```python
from build123d import *

# Parameters (mm, degrees)
F0_W     = 89.4973501563
F0_H     = 37.3169183731
F1_DEPTH = 76.2
F2_R     = 5.08
F3_SIZE  = 25.4
F4_T     = -2.54
F6_D     = 6.35


# Not quite as in the source:
# - a shell that OpenCascade refuses in one call is made with other operations: the cavity is built on its own and cut out


with BuildPart() as f1:
    # F0 (on Front) → F1 (new body)
    with BuildSketch(Plane.XZ):
        with Locations((0.0334233046, 18.6584591866)):
            Rectangle(F0_W, F0_H)
    extrude(amount=F1_DEPTH)

    # F2
    f2_edges = [f1.edges().sort_by_distance(p)[0] for p in [
        (44.782098, -38.1, 37.316918),
        (0.033423, -76.2, 37.316918),
        (-44.715252, -38.1, 37.316918),
        (0.033423, 0, 37.316918),
    ]]
    fillet(f2_edges, radius=F2_R)

    # F3
    f3_edges = [f1.edges().sort_by_distance(p)[0] for p in [
        (-44.715252, -38.1, 0),
        (0.033423, 0, 0),
        (44.782098, -38.1, 0),
        (0.033423, -76.2, 0),
    ]]
    chamfer(f3_edges, length=F3_SIZE)

    # F4: a shell. OpenCascade refuses it in one call, so the cavity is built on its own and cut out:
    # the body offset inwards by the wall thickness, plus a prism from it out through each open face.
    f4_core = offset(f1.part, amount=F4_T, mode=Mode.PRIVATE)
    f4_exits = [f4_core.faces().sort_by_distance(p)[0] for p in [
        (0.033423, -38.1, 34.776918),
    ]]
    add(f4_core, mode=Mode.SUBTRACT)
    extrude(f4_exits, amount=-F4_T, mode=Mode.SUBTRACT)

    # F6 (through all)
    with Locations(Plane.XY.offset(2.54)):
        with Locations((0.0334233046, -40.5182316899)):
            Hole(F6_D / 2)


solid = f1.part
```
Geometry check sheet. Reference: the model listing, model coordinates, mm. A direction names the side the tool comes from. Give positions to 0.01 mm unless a question says otherwise; leave off trailing zeros. Order: outer loops, then holes, each group sorted by start corner. A loop starts at its lowest first (then second) coordinate and runs counter-clockwise, first axis right, second up. Notation, with made-up numbers: (67, 15.5) - (93, 15.5) arc R27 ccw to (93, 32.5) - close; hole circle Ø8 at (-3.75, -0.5). An arc over 180 degrees is marked (long way). Write item = value, one per line. Start each with the question number.
1) Section check B-B (z = 5). Enter the section's corners in (x, y).
2) Section check D-D (z = 17). Enter the section's corners in (x, y).
3) Section check C-C (y = -67). Enter the section's corners in (x, z).
4) Gauge pin test, flat ends, axial feed: pin 1 Ø6 at (x, z) = (9, 12) entering from -Y; pin 2 Ø1 at (y, z) = (-50.5, 8.5) entering from +X; pin 3 Ø1.3 at (y, z) = (-25.5, 35.5) entering from +X; pin 4 Ø5 at (x, y) = (0.03, -40.52) entering from +Z. Record the tip position at first contact, or that the pin passes through.
5) Draft check along X on faces 1 (the flat face through (42.242, -38, 29)), 2 (the cylindrical face through (43.333, -38.633, 35.789)), 3 (the flat face through (-34.66, -37.567, 15.344)). Enter one of: released by +X, released by -X, zero draft, split by the parting line, or undercut.
6) Access from +Z, -Z, +X, -X, +Y, -Y to the whole of each face (thin tool, end or side, straight path). Record for faces 4 (the cylindrical face through (-41.451, -38.598, 34.013)), 5 (the flat face through (-0.6, -66.5, 15.7)), 6 (the flat face through (0, -35, 2.54)).
7) Scan lines: L1, parallel to X at y = -32.5, z = 29.5; L2, parallel to Y at x = 36, z = 27; L3, parallel to Z at x = -3.5, y = -34. Record each from-to range of solid material in increasing order.
8) Section check A-A (x = -16.5). Enter the section's corners in (y, z), then the cut area to 3 significant figures.
Geometry check:
q1.outline = (-24.32, -55.8) - (24.38, -55.8) - (24.38, -20.4) - (-24.32, -20.4) - close; hole (-20.72, -52.21) - (20.79, -52.21) - (20.79, -23.99) - (-20.72, -23.99) - close
q2.outline = (-36.32, -67.8) - (36.38, -67.8) - (36.38, -8.4) - (-36.32, -8.4) - close; hole (-32.72, -64.21) - (32.79, -64.21) - (32.79, -11.99) - (-32.72, -11.99) - close
q3.outline = (-44.72, 25.4) - (-35.52, 16.2) - (35.58, 16.2) - (44.78, 25.4) - (44.78, 32.24) arc R5.08 ccw to (39.7, 37.32) - (39.7, 34.78) arc R2.54 cw to (42.24, 32.24) - (42.24, 26.45) - (35.58, 19.79) - (-35.52, 19.79) - (-42.18, 26.45) - (-42.18, 32.24) arc R2.54 cw to (-39.64, 34.78) - (-39.64, 37.32) arc R5.08 ccw to (-44.72, 32.24) - close
q4.pin_1 = -65.8
q4.pin_2 = 28.38
q4.pin_3 = 44.06
q4.pin_4 = through
q5.face_1 = undercut
q5.face_2 = released by +X
q5.face_3 = released by -X
q6.face_4 = none
q6.face_5 = -Z, +X, -X, -Y
q6.face_6 = +Z
q7.L1 = -44.72 to -42.18, 42.24 to 44.78
q7.L2 = -76.2 to -73.66, -2.54 to 0
q7.L3 = 0 to 2.54
q8.outline = (-76.2, 25.4) - (-50.8, 0) - (-25.4, 0) - (0, 25.4) - (0, 32.24) arc R5.08 ccw to (-5.08, 37.32) - (-5.08, 34.78) arc R2.54 cw to (-2.54, 32.24) - (-2.54, 26.45) - (-26.45, 2.54) - (-49.75, 2.54) - (-73.66, 26.45) - (-73.66, 32.24) arc R2.54 cw to (-71.12, 34.78) - (-71.12, 37.32) arc R5.08 ccw to (-76.2, 32.24) - close
q8.area = 301 mm2
